Source: CAD feature listing. Evaluate the final solid. Frame: model axes, mm. A direction names the side the tool comes from. Give positions to 0.01 mm unless a question says otherwise; leave off trailing zeros. Loops run counter-clockwise (first coordinate to the right, second up) from the corner with the lowest first, then second, coordinate; pieces in that order, holes last. Notation, with made-up numbers: (71, 48) -> (103, 48) arc R19 ccw to (103, 85) -> close; hole circle Ø11 at (28, 31.5). An arc over 180 degrees is marked (long way). Put each result on its own line as item: value.
```python
from build123d import *

# Parameters (mm, degrees)
SKETCH2_W               = 47.573593128
SKETCH2_H               = 35
BOSS_EXTRUDE1_DEPTH     = 90
CUT_EXTRUDE1_DEPTH      = 40
CUT_EXTRUDE1_DEPTH_BACK = 40
SKETCH4_W               = 55
SKETCH4_H               = 35
CUT_EXTRUDE2_DEPTH      = 5


with BuildPart() as part:
    # Sketch2 → Boss-Extrude1 (new body)
    with BuildSketch(Plane(origin=(0, 0, 0), x_dir=(0, 0, -1), z_dir=(1, 0, 0))):
        Polygon((-23.786796564, 17.5), (-66.213203436, -17.5), (-23.786796564, -17.5), align=None)
        Rectangle(SKETCH2_W, SKETCH2_H)
        Polygon((-21.990568975, 12.5), (-23.786796564, 11.018187839), (-23.786796564, -17.5), (18.786796564, -17.5), (18.786796564, 12.5), align=None)
        Polygon((-23.786796564, -17.5), (-23.786796564, 11.018187839), (-58.356060578, -17.5), align=None)
    extrude(amount=-BOSS_EXTRUDE1_DEPTH)

    # Sketch3 → Cut-Extrude1 (cut, two sides: drawn at the far end of the back side and taken through both)
    with BuildSketch(Plane.ZY.offset(45).offset(-CUT_EXTRUDE1_DEPTH_BACK)):
        Polygon((-18.786796564, -17.5), (-18.786796564, 12.5), (21.990568975, 12.5), (58.356060578, -17.5), align=None)
    extrude(amount=CUT_EXTRUDE1_DEPTH + CUT_EXTRUDE1_DEPTH_BACK, mode=Mode.SUBTRACT)

    # Sketch4 → Cut-Extrude2 (cut)
    with BuildSketch(Plane(origin=(0, 22.08978209, 18.223140496), x_dir=(1, 0, 0), z_dir=(0, 0.77138921583987, 0.6363636363636365))):
        with Locations((-52.5, -34.712514713)):
            Rectangle(SKETCH4_W, SKETCH4_H)
    extrude(amount=-CUT_EXTRUDE2_DEPTH, mode=Mode.SUBTRACT)


solid = part.part
```
(1) Section C-C on x = -17.5. Return loops of the section in (y, z).
Calculated:
outline: (-17.5, -23.79) -> (17.5, -23.79) -> (17.5, 23.79) -> (-17.5, 66.21) -> (-17.5, 58.36) -> (12.5, 21.99) -> (12.5, -18.79) -> (-17.5, -18.79) -> close
(2) Draft query along X for faces 4 (the flat face through (-44, 12.5, 1)), 5 (the flat face through (-24, 0, 45)), 6 (the flat face through (0, 0, 12)), 7 (the flat face through (-25, -2, 44)). Return one class per face: released by +X, released by -X, zero draft, split by the parting line, or undercut.
Calculated:
face 4: undercut
face 5: zero draft
face 6: released by +X
face 7: undercut
(3) Section B-B on z = -3. Return loops of the section in (x, y).
Calculated:
outline: (-90, -17.5) -> (-85, -17.5) -> (-85, 12.5) -> (-5, 12.5) -> (-5, -17.5) -> (0, -17.5) -> (0, 17.5) -> (-90, 17.5) -> close
(4) First-contact query: P1, Ø20.5, axis at x = -52.5, z = 8, coming from the -Y side; P2, Ø15, axis at x = -32.5, y = -7, coming from the +Z side. Flat tips, straight axial feed; report the tip coordinate or a pass-through.
Calculated:
P1: stops at y = 12.5
P2: stops at z = 62.58
(5) Section A-A on x = -78. Return loops of the section in (y, z).
Calculated:
outline: (-17.5, -23.79) -> (17.5, -23.79) -> (17.5, 23.79) -> (11.14, 31.5) -> (7.28, 28.32) -> (12.5, 21.99) -> (12.5, -18.79) -> (-17.5, -18.79) -> close; (-17.5, 58.36) -> (-14.99, 55.32) -> (-11.14, 58.5) -> (-17.5, 66.21) -> close
(6) Reachability of faces 1 (the flat face through (-52.88, -13.04, 56.93)), 2 (the flat face through (-44, -3, -18.787)), 3 (the flat face through (-52.88, 9.23, 29.93)) from +Z, -Z, +X, -X, +Y, -Y: full face, straight path, thin tool, end or side. Return the list, or none.
Calculated:
face 1: +Y
face 2: -Y
face 3: +Z, -Y
(7) Section D-D on z = 49.5. Return loops of the section in (x, y), then the cut area to 3 significant figures.
Calculated:
outline: (-90, -17.5) -> (-85, -17.5) -> (-85, -10.19) -> (-80, -10.19) -> (-80, -3.71) -> (-90, -3.71) -> close; (-25, -10.19) -> (-5, -10.19) -> (-5, -17.5) -> (0, -17.5) -> (0, -3.71) -> (-25, -3.71) -> close
area: 300 mm²
(8) Line query: probe 1 along X at (y, z) = (-10, 49); probe 2 along Z at (x, y) = (-83.5, -12); probe 3 along Z at (x, y) = (-24, -14.5). Output: solid intervals per line, ascending. Write a range as from..to.
Calculated:
probe 1: x = -90..-85, -5..0
probe 2: z = -23.79..-18.79, 51.69..59.55
probe 3: z = -23.79..-18.79, 54.72..62.58
